```python
from build123d import *

# Parameters (mm, degrees)
SKETCH1_W               = 138
SKETCH1_H               = 28
BOSS_EXTRUDE1_DEPTH     = 1.5
SKETCH2_W               = 28
SKETCH2_H               = 59
BOSS_EXTRUDE2_DEPTH     = 1.5
FILLET1_R               = 1
FILLET2_R               = 1
FILLET5_R               = 10
SKETCH3_R               = 1.25
CUT_EXTRUDE1_DEPTH      = 15
CUT_EXTRUDE1_DEPTH_BACK = 15
SKETCH4_W               = 28
SKETCH4_H               = 59
BOSS_EXTRUDE3_DEPTH     = 1.5
FILLET6_R               = 1
FILLET7_R               = 1
SKETCH5_R               = 1.5
CUT_EXTRUDE3_DEPTH      = 1.5
CUT_EXTRUDE3_DEPTH_BACK = 31.5
FILLET10_R              = 10
FILLET11_R              = 10


with BuildPart() as part:
    # Sketch1 → Boss-Extrude1 (new body)
    with BuildSketch(Plane(origin=(0, 0, 0), x_dir=(1, 0, 0), z_dir=(0, 1, 0))):
        with Locations((69, 14)):
            Rectangle(SKETCH1_W, SKETCH1_H)
    extrude(amount=BOSS_EXTRUDE1_DEPTH)

    # Sketch2 → Boss-Extrude2 (add)
    with BuildSketch(Plane(origin=(0, 0, 0), x_dir=(0, 0, -1), z_dir=(1, 0, 0))):
        with Locations((14, 29.5)):
            Rectangle(SKETCH2_W, SKETCH2_H)
    extrude(amount=-BOSS_EXTRUDE2_DEPTH)

    # Fillet1
    fillet1_edges = [part.edges().sort_by_distance(p)[0] for p in [
        (0, 1.5, -14),
    ]]
    fillet(fillet1_edges, radius=FILLET1_R)

    # Fillet2
    fillet2_edges = [part.edges().sort_by_distance(p)[0] for p in [
        (-1.5, 0, -14),
    ]]
    fillet(fillet2_edges, radius=FILLET2_R)

    # Fillet5
    fillet5_edges = [part.edges().sort_by_distance(p)[0] for p in [
        (-0.75, 59, 0),
        (-0.75, 59, -28),
    ]]
    fillet(fillet5_edges, radius=FILLET5_R)

    # Sketch3 → Cut-Extrude1 (cut, two sides)
    with BuildSketch(Plane(origin=(0, 0, 0), x_dir=(0, 0, -1), z_dir=(1, 0, 0))) as cut_extrude1_sk:
        with Locations((14, 52.5)):
            Circle(SKETCH3_R)
        with Locations((6.5, 45)):
            Circle(SKETCH3_R)
        with Locations((14, 45)):
            Circle(SKETCH3_R)
        with Locations((21.5, 45)):
            Circle(SKETCH3_R)
        with Locations((14, 37.5)):
            Circle(SKETCH3_R)
    extrude(amount=CUT_EXTRUDE1_DEPTH, mode=Mode.SUBTRACT)
    extrude(cut_extrude1_sk.sketch, amount=-CUT_EXTRUDE1_DEPTH_BACK, mode=Mode.SUBTRACT)

    # Sketch4 → Boss-Extrude3 (add)
    with BuildSketch(Plane(origin=(138, 0, 0), x_dir=(0, 0, -1), z_dir=(1, 0, 0))):
        with Locations((14, 29.5)):
            Rectangle(SKETCH4_W, SKETCH4_H)
    extrude(amount=BOSS_EXTRUDE3_DEPTH)

    # Fillet6
    fillet6_edges = [part.edges().sort_by_distance(p)[0] for p in [
        (139.5, 0, -14),
    ]]
    fillet(fillet6_edges, radius=FILLET6_R)

    # Fillet7
    fillet7_edges = [part.edges().sort_by_distance(p)[0] for p in [
        (138, 1.5, -14),
    ]]
    fillet(fillet7_edges, radius=FILLET7_R)

    # Sketch5 → Cut-Extrude3 (cut, two sides)
    with BuildSketch(Plane(origin=(139.5, 0, 0), x_dir=(0, 0, -1), z_dir=(1, 0, 0))) as cut_extrude3_sk:
        with Locations((14, 45)):
            Circle(SKETCH5_R)
    extrude(amount=CUT_EXTRUDE3_DEPTH, mode=Mode.SUBTRACT)
    extrude(cut_extrude3_sk.sketch, amount=-CUT_EXTRUDE3_DEPTH_BACK, mode=Mode.SUBTRACT)

    # Fillet10
    fillet10_edges = [part.edges().sort_by_distance(p)[0] for p in [
        (138.75, 59, -28),
    ]]
    fillet(fillet10_edges, radius=FILLET10_R)

    # Fillet11
    fillet11_edges = [part.edges().sort_by_distance(p)[0] for p in [
        (138.75, 59, 0),
    ]]
    fillet(fillet11_edges, radius=FILLET11_R)


solid = part.part
```
Input: part model. Units: mm. Frame: model coordinates. A direction names the side the tool comes from. Round coordinates to 2 decimals unless told otherwise and drop trailing zeros. Loops run counter-clockwise (first coordinate to the right, second up) from the corner with the lowest first, then second, coordinate; pieces in that order, holes last. Notation, with made-up numbers: (-27.75, 7) -> (-11.75, 7) arc R18 ccw to (-11.75, 15) -> close; hole circle Ø8 at (-30, 16.5). An arc over 180 degrees is marked (long way). Use one line per item in the form item = value. Start each with the question number.
Item 1: Section query D-D on z = -6.5. Return the cut outline in (x, y), then the cut area to 3 significant figures.
Item 2: Section query A-A on z = -14. Return the cut outline in (x, y).
Item 3: Material intervals for L1, parallel to X at y = 17, z = -15.75; L2, parallel to Y at x = -0.55, z = -14; L3, parallel to Y at x = -1.1, z = -14, sorted ascending. Write a range as from..to.
Item 4: Section query C-C on y = 29. Return the cut outline in (x, z).
Item 5: Section query B-B on y = 37.5. Return the cut outline in (x, z), then the cut area to 4 significant figures.
Item 6: Set-up query: faces 4 (the face through (-0.74, 46.24, -21.34)), 5 (the face through (138.76, 43.536, -13.675)), 6 (the face through (0, 31, -14)). Return all of +Z, -Z, +X, -X, +Y, -Y with unobstructed straight access to the full face (end or side cutting, diameter ignored); none if empty.
Item 7: Mould query, pull axis Y, two halves, no side actions, for faces 1 (the face through (68, 1.5, -14)), 2 (the face through (139.5, 30, -14)), 3 (the face through (-0.74, 53.74, -13.84)). Classes: pulls with the +Y half, pulls with the -Y half, needs draft (parallel to the pull), parting line crosses it, or undercut.
Item 8: Contact query for flat-ended pins moving along their axis: pin 1 Ø3 at (x, z) = (67.5, -16.5) entering from +Y; pin 2 Ø1.5 at (y, z) = (37.5, -14) entering from -X; pin 3 Ø8 at (x, y) = (95, 6.5) entering from +Z. Output: stop coordinate, or through.
Ans:
q1.outline = (-1.5, 1) arc R1 ccw to (-0.5, 0) -> (138.5, 0) arc R1 ccw to (139.5, 1) -> (139.5, 58.37) -> (138, 58.37) -> (138, 2.5) arc R1 cw to (137, 1.5) -> (1, 1.5) arc R1 cw to (0, 2.5) -> (0, 43.75) -> (-1.5, 43.75) -> close; (-1.5, 46.25) -> (0, 46.25) -> (0, 58.37) -> (-1.5, 58.37) -> close
q1.area = 378 mm^2
q2.outline = (-1.5, 1) arc R1 ccw to (-0.5, 0) -> (138.5, 0) arc R1 ccw to (139.5, 1) -> (139.5, 43.5) -> (138, 43.5) -> (138, 2.5) arc R1 cw to (137, 1.5) -> (1, 1.5) arc R1 cw to (0, 2.5) -> (0, 36.25) -> (-1.5, 36.25) -> close; (-1.5, 38.75) -> (0, 38.75) -> (0, 43.75) -> (-1.5, 43.75) -> close; (-1.5, 46.25) -> (0, 46.25) -> (0, 51.25) -> (-1.5, 51.25) -> close; (-1.5, 53.75) -> (0, 53.75) -> (0, 59) -> (-1.5, 59) -> close; (138, 46.5) -> (139.5, 46.5) -> (139.5, 59) -> (138, 59) -> close
q3.L1 = -1.5..0, 138..139.5
q3.L2 = 0..36.25, 38.75..43.75, 46.25..51.25, 53.75..59
q3.L3 = 0.2..36.25, 38.75..43.75, 46.25..51.25, 53.75..59
q4.outline = (-1.5, -28) -> (0, -28) -> (0, 0) -> (-1.5, 0) -> close; (138, -28) -> (139.5, -28) -> (139.5, 0) -> (138, 0) -> close
q5.outline = (-1.5, -28) -> (0, -28) -> (0, -15.25) -> (-1.5, -15.25) -> close; (-1.5, -12.75) -> (0, -12.75) -> (0, 0) -> (-1.5, 0) -> close; (138, -28) -> (139.5, -28) -> (139.5, 0) -> (138, 0) -> close
q5.area = 80.25 mm^2
q6.face_4 = -X
q6.face_5 = +X
q6.face_6 = +Z, -Z, +Y
q7.face_1 = pulls with the +Y half
q7.face_2 = needs draft
q7.face_3 = undercut
q8.pin_1 = 1.5
q8.pin_2 = 138
q8.pin_3 = through
